Here's how the part is built. I have some questions about the finished solid (model axes, mm). Face numbers are marked on the shaded views. A direction names the side the tool comes from. Round coordinates to 2 decimals unless told otherwise and drop trailing zeros. Loops run counter-clockwise (first coordinate to the right, second up) from the corner with the lowest first, then second, coordinate; pieces in that order, holes last. Notation, with made-up numbers: (-34, -7.5) - (-2, -7.5) arc R21 cw to (-2, 19.5) - close; hole circle Ø1 at (12, 16). An arc over 180 degrees is marked (long way). Return JSON: item names as keys, results as strings. Group by question number.
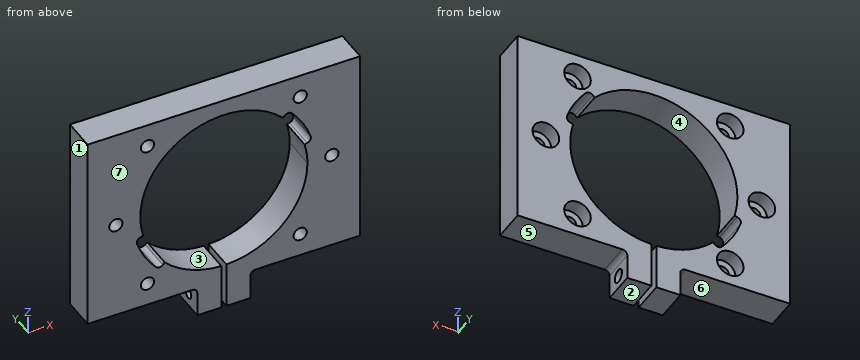
```python
from build123d import *

# Parameters (mm, degrees)
SKETCH1_W           = 82
SKETCH1_H           = 60
SKETCH1_R           = 1.999999999
SKETCH1_R_2         = 2.000000001
SKETCH1_R_3         = 1.999999998
SKETCH1_R_4         = 2.000000002
BOSS_EXTRUDE1_DEPTH = 10
SKETCH2_W           = 16
SKETCH2_H           = 9
BOSS_EXTRUDE2_DEPTH = 10
SKETCH3_W           = 1.5
SKETCH3_H           = 14
CUT_EXTRUDE1_DEPTH  = 10
SKETCH4_R           = 2
CUT_EXTRUDE2_DEPTH  = 7.25
SKETCH5_R           = 1.6
CUT_EXTRUDE3_DEPTH  = 10
SKETCH7_R           = 4.000000002
SKETCH7_R_2         = 4.000000001
SKETCH7_R_3         = 4
SKETCH7_R_4         = 3.999999999
SKETCH7_R_5         = 3.999999998
CUT_EXTRUDE4_DEPTH  = 4.5
FILLET1_R           = 1.5


with BuildPart() as part:
    # Sketch1 → Boss-Extrude1 (new body)
    with BuildSketch(Plane(origin=(0, 76, 0), x_dir=(1, 0, 0), z_dir=(0, 1, 0))):
        Rectangle(SKETCH1_W, SKETCH1_H)
        with Locations(Location((-22.980970387, -22.98097039, 0), (0, 0, 270))):
            Circle(SKETCH1_R, mode=Mode.SUBTRACT)
        with Locations(Location((-32.5, -2e-09, 0), (0, 0, 270))):
            Circle(SKETCH1_R_2, mode=Mode.SUBTRACT)
        with Locations(Location((22.98097039, -22.980970387, 0), (0, 0, 270))):
            Circle(SKETCH1_R_3, mode=Mode.SUBTRACT)
        with BuildLine():
            ThreePointArc((-20.534900496, 18.291196287), (-19.458102274, 18.792869946), (-18.354154843, 18.354154843))
            Line((-18.354154843, 18.354154843), (-17.783735547, 17.783735547))
            ThreePointArc((-17.783735547, 17.783735547), (9.624488324, 23.235570243), (25.15, 0))
            ThreePointArc((25.15, 0), (24.934838264, -3.282733734), (24.293034531, -6.509298984))
            Line((24.293034531, -6.509298984), (25.072241781, -6.718086938))
            ThreePointArc((25.072241781, -6.718086938), (26.00415392, -7.454775906), (26.108090898, -8.638147351))
            ThreePointArc((26.108090898, -8.638147351), (23.815698604, -13.75), (20.534900496, -18.291196287))
            ThreePointArc((20.534900496, -18.291196287), (19.458102274, -18.792869946), (18.354154843, -18.354154843))
            Line((18.354154843, -18.354154843), (17.783735547, -17.783735547))
            ThreePointArc((17.783735547, -17.783735547), (-12.575, -21.780538905), (-24.293034531, 6.509298984))
            Line((-24.293034531, 6.509298984), (-25.072241781, 6.718086938))
            ThreePointArc((-25.072241781, 6.718086938), (-26.00415392, 7.454775906), (-26.108090898, 8.638147351))
            ThreePointArc((-26.108090898, 8.638147351), (-23.815698604, 13.75), (-20.534900496, 18.291196287))
        make_face(mode=Mode.SUBTRACT)
        with Locations(Location((-22.98097039, 22.980970387, 0), (0, 0, 270))):
            Circle(SKETCH1_R_4, mode=Mode.SUBTRACT)
        with Locations(Location((32.5, 2e-09, 0), (0, 0, 270))):
            Circle(SKETCH1_R, mode=Mode.SUBTRACT)
        with Locations(Location((22.980970387, 22.98097039, 0), (0, 0, 270))):
            Circle(SKETCH1_R_2, mode=Mode.SUBTRACT)
    extrude(amount=BOSS_EXTRUDE1_DEPTH)

    # Sketch2 → Boss-Extrude2 (add)
    with BuildSketch(Plane(origin=(0, 86, 0), x_dir=(1, 0, 0), z_dir=(0, 1, 0))):
        with Locations((0, 34.5)):
            Rectangle(SKETCH2_W, SKETCH2_H)
    extrude(amount=-BOSS_EXTRUDE2_DEPTH)

    # Sketch3 → Cut-Extrude1 (cut)
    with BuildSketch(Plane(origin=(0, 86, 0), x_dir=(1, 0, 0), z_dir=(0, 1, 0))):
        with Locations((0, 32)):
            Rectangle(SKETCH3_W, SKETCH3_H)
    extrude(amount=-CUT_EXTRUDE1_DEPTH, mode=Mode.SUBTRACT)

    # Sketch4 → Cut-Extrude2 (cut)
    with BuildSketch(Plane(origin=(8, 0, 0), x_dir=(0, 0, -1), z_dir=(1, 0, 0))):
        with Locations((35, 81)):
            Circle(SKETCH4_R)
    extrude(amount=-CUT_EXTRUDE2_DEPTH, mode=Mode.SUBTRACT)

    # Sketch5 → Cut-Extrude3 (cut)
    with BuildSketch(Plane(origin=(-0.75, 0, 0), x_dir=(0, 0, -1), z_dir=(1, 0, 0))):
        with Locations((35, 81)):
            Circle(SKETCH5_R)
    extrude(amount=-CUT_EXTRUDE3_DEPTH, mode=Mode.SUBTRACT)

    # Sketch7 → Cut-Extrude4 (cut)
    with BuildSketch(Plane(origin=(0, 86, 0), x_dir=(1, 0, 0), z_dir=(0, 1, 0))):
        with Locations(Location((-22.98097039, 22.980970387, 0), (0, 0, 270))):
            Circle(SKETCH7_R)
        with Locations(Location((22.980970387, 22.98097039, 0), (0, 0, 270))):
            Circle(SKETCH7_R_2)
        with Locations(Location((32.5, 0, 0), (0, 0, 270))):
            Circle(SKETCH7_R_3)
        with Locations(Location((-32.5, 0, 0), (0, 0, 270))):
            Circle(SKETCH7_R_3)
        with Locations(Location((-22.980970387, -22.98097039, 0), (0, 0, 270))):
            Circle(SKETCH7_R_4)
        with Locations(Location((22.98097039, -22.980970387, 0), (0, 0, 270))):
            Circle(SKETCH7_R_5)
    extrude(amount=-CUT_EXTRUDE4_DEPTH, mode=Mode.SUBTRACT)

    # Fillet1
    fillet1_edges = [part.edges().sort_by_distance(p)[0] for p in [
        (8, 81, -30),
        (-8, 81, -30),
    ]]
    fillet(fillet1_edges, radius=FILLET1_R)


solid = part.part
```
Q1. For the marked faces 5, 6 and 7, which set-ups out of +Z, -Z, +X, -X, +Y, -Y let a thin tool reach every point of the face, with its end or its side?
Q2. Will these pins go through, and if not, where does the flat tip stop? pin 1 Ø6.5 at (x, z) = (22.98, 22.98) entering from +Y; pin 2 Ø1.5 at (x, y) = (16.5, 82.5) entering from -Z; pin 3 Ø4 at (y, z) = (81, -35) entering from -X.
Q3. Please list where these lines run through material, in increasing order: line 1 (Z direction, x = 1, y = 78.5); line 2 (X direction, y = 79, z = 0.5); line 3 (X direction, y = 84.25, z = 2.5).
Q4. Imagine slicing it at D-D, the plane x = -15.5. List the corners of the cut face in (y, z) for me, and give its area (3 significant figures).
Q5. Imagine slicing it at B-B, the plane z = -15. List the corners of the cut face in (x, y) for me.
Q6. Imagine slicing it at A-A, the plane x = 32.5. List the corners of the cut face in (y, z) for me, and give its area (3 significant figures).
Q7. Imagine slicing it at C-C, the plane y = 85. Give the number of separate pieces and of enclosed holes in the cut face, and give its area (3 significant figures).
Q8. If we mould it in two halves opening along Z, with no side actions, what happens to the marked faces 1, 2, 3 and 4? For each: +Z half, -Z half, draft (parallel to the pull), parting line (faces both ways), or undercut.
Output values:
{
 "1": {"face 5": "-Z, +X, +Y, -Y", "face 6": "-Z, -X, +Y, -Y", "face 7": "+Z, -Z, +X, -X, -Y"},
 "2": {"pin 1": "stops at y = 81.5", "pin 2": "stops at z = -30", "pin 3": "stops at x = -8"},
 "3": {"line 1": "z = -39 to -25.13, 25.13 to 30", "line 2": "x = -41 to -34.44, -30.56 to -25.15, 25.15 to 30.56, 34.44 to 41", "line 3": "x = -41 to -35.62, -29.38 to -25.03, 25.03 to 29.38, 35.62 to 41"},
 "4": {"outline": "(76, -30) - (86, -30) - (86, -19.81) - (76, -19.81) - close; (76, 19.81) - (86, 19.81) - (86, 30) - (76, 30) - close", "area": "204 mm^2"},
 "5": {"outline": "(-41, 76) - (-23.05, 76) - (-23.05, 86) - (-41, 86) - close; (20.19, 76) - (41, 76) - (41, 86) - (20.19, 86) - close"},
 "6": {"outline": "(76, -30) - (86, -30) - (86, -4) - (81.5, -4) - (81.5, -2) - (76, -2) - close; (76, 2) - (81.5, 2) - (81.5, 4) - (86, 4) - (86, 30) - (76, 30) - close", "area": "542 mm^2"},
 "7": {"separate pieces": "1", "enclosed holes": "6", "area": "2,690 mm^2"},
 "8": {"face 1": "draft", "face 2": "-Z half", "face 3": "undercut", "face 4": "undercut"}
}
